Input: part model. Units: mm. Frame: model coordinates. A direction names the side the tool comes from. Round coordinates to 2 decimals unless told otherwise and drop trailing zeros. Loops run counter-clockwise (first coordinate to the right, second up) from the corner with the lowest first, then second, coordinate; pieces in that order, holes last. Notation, with made-up numbers: (54, -9) -> (99, -9) arc R13 ccw to (99, 2) -> close; hole circle Ø7 at (23.5, 79.5). An arc over 180 degrees is marked (long way). Answer as a JSON object with one key per item and string values. Group by question number.
Item 1: Pin query (flat end, axial travel): pin 1 (2.5 mm diameter, centred on y = 3.5, z = 11.5, fed in from -X); pin 2 (2 mm diameter, centred on x = -3, y = 3, fed in from +Z); pin 3 (1.6 mm diameter, centred on y = 3, z = -1.5, fed in from +X) (3 decimals). Return the tip coordinate at first contact, or that it passes through.
Item 2: Section query B-B on x = 0. Return loops of the section in (y, z), and give its area (3 significant figures).
Item 3: Material intervals for line 1 (X direction, y = -10.4, z = 17); line 2 (Y direction, x = 0.75, z = -4); line 3 (X direction, y = 4, z = -7.25) (3 decimals), sorted ascending. Write a range as [from, to].
Item 4: Draft query along Z for faces 1 (the flat face through (0, 0, 1)), 2 (the cylindrical face through (5.68, 3.97, 18.25)), 3 (the flat face through (3.9, 3, 11)). Return one class per face: released by +Z, released by -Z, zero draft, split by the parting line, or undercut.
Item 5: Section query A-A on y = 2. Return loops of the section in (x, z) (3 decimals), and give its area (3 significant figures).
Item 6: Section query D-D on y = -11. Return loops of the section in (x, z), and give its area (3 significant figures).
Item 7: Section query C-C on z = 3.25. Return loops of the section in (x, y) (3 decimals), and give its area (3 significant figures).
Item 8: Set-up query: faces 4 (the flat face through (-5, 2.7, 16)), 5 (the cylindrical face through (-4.4, 2.56, 7.83)), 6 (the flat face through (-4.875, 3, 0)). Return all of +Z, -Z, +X, -X, +Y, -Y with unobstructed straight access to the full face (end or side cutting, diameter ignored); none if empty.
from build123d import *

# Parameters (mm, degrees)
BOSS_EXTRUDE1_DEPTH = 5.2
SKETCH5_W           = 7.8
SKETCH5_H           = 5.2
BOSS_EXTRUDE2_DEPTH = 17
SKETCH6_R           = 3.9
BOSS_EXTRUDE3_DEPTH = 18.5
BOSS_EXTRUDE4_DEPTH = 2.5
SKETCH8_R           = 1.6
CUT_EXTRUDE1_DEPTH  = 5


with BuildPart() as part:
    # Sketch3 → Boss-Extrude1 (new body)
    with BuildSketch(Plane(origin=(0, 0, 0), x_dir=(1, 0, 0), z_dir=(0, 1, 0))):
        with BuildLine():
            Line((-4.875, 7.545253061), (-4.875, -7.545253061))
            ThreePointArc((-4.875, -7.545253061), (0, -8.983121325), (4.875, -7.545253061))
            Line((4.875, -7.545253061), (4.875, 7.545253061))
            ThreePointArc((4.875, 7.545253061), (0, 8.983121325), (-4.875, 7.545253061))
        make_face()
    extrude(amount=BOSS_EXTRUDE1_DEPTH)

    # Sketch5 → Boss-Extrude2 (add)
    with BuildSketch(Plane.XY):
        with Locations((0, 2.6)):
            Rectangle(SKETCH5_W, SKETCH5_H)
    extrude(amount=BOSS_EXTRUDE2_DEPTH)

    # Sketch6 → Boss-Extrude3 (add)
    with BuildSketch(Plane(origin=(0, 5.2, 0), x_dir=(1, 0, 0), z_dir=(0, 1, 0))):
        with Locations(Location((0, -17, 0), (0, 0, 270))):
            Circle(SKETCH6_R)
    extrude(amount=-BOSS_EXTRUDE3_DEPTH)

    # Sketch7 → Boss-Extrude4 (add)
    with BuildSketch(Plane(origin=(0, 5.2, 0), x_dir=(1, 0, 0), z_dir=(0, 1, 0))):
        with BuildLine():
            Line((-4.4, -14), (4.4, -14))
            ThreePointArc((4.4, -14), (6.167766953, -14.732233047), (6.9, -16.5))
            Line((6.9, -16.5), (6.9, -17))
            ThreePointArc((6.9, -17), (5.65, -18.25), (4.4, -17))
            Line((4.4, -17), (-4.4, -17))
            ThreePointArc((-4.4, -17), (-5.65, -18.25), (-6.9, -17))
            Line((-6.9, -17), (-6.9, -16.5))
            ThreePointArc((-6.9, -16.5), (-6.167766953, -14.732233047), (-4.4, -14))
        make_face()
    extrude(amount=-BOSS_EXTRUDE4_DEPTH)

    # Sketch8 → Cut-Extrude1 (cut)
    with BuildSketch(Plane.XZ.offset(13.3)):
        with Locations(Location((0, 17, 0), (0, 0, 270))):
            Circle(SKETCH8_R)
    extrude(amount=-CUT_EXTRUDE1_DEPTH, mode=Mode.SUBTRACT)


solid = part.part
Solved:
{
 "1": {"pin 1": "x = -3.9", "pin 2": "z = 20.35", "pin 3": "x = 4.875"},
 "2": {"outline": "(-13.3, 13.1) -> (0, 13.1) -> (0, -8.98) -> (5.2, -8.98) -> (5.2, 20.9) -> (-13.3, 20.9) -> (-13.3, 18.6) -> (-8.3, 18.6) -> (-8.3, 15.4) -> (-13.3, 15.4) -> close", "area": "243 mm²"},
 "3": {"line 1": "[-3.9, -1.6], [1.6, 3.9]", "line 2": "[0, 5.2]", "line 3": "[-4.875, 4.875]"},
 "4": {"face 1": "zero draft", "face 2": "released by +Z", "face 3": "undercut"},
 "5": {"outline": "(-4.875, -7.545) arc R8.983 ccw to (4.875, -7.545) -> (4.875, 7.545) arc R8.983 ccw to (3.9, 8.092) -> (3.9, 17) arc R3.9 ccw to (-3.9, 17) -> (-3.9, 8.092) arc R8.983 ccw to (-4.875, 7.545) -> close", "area": "255 mm²"},
 "6": {"outline": "circle Ø7.8 at (0, 17); hole circle Ø3.2 at (0, 17)", "area": "39.7 mm²"},
 "7": {"outline": "(-4.875, 0) -> (4.875, 0) -> (4.875, 5.2) -> (-4.875, 5.2) -> close", "area": "50.7 mm²"},
 "8": {"face 4": "+Z, -X, -Y", "face 5": "-X, +Y, -Y", "face 6": "-Z, -X, +Y, -Y"}
}
